from build123d import *

# Parameters (mm, degrees)
F1_DEPTH = 63.5
F0_W     = 25.4
F0_H     = 19.05
F2_DEPTH = 25.4
F3_DEPTH = 7.9375
F5_R     = 6.35


with BuildPart() as f1:
    # F0 (on Front) → F1 (new body, symmetric)
    with BuildSketch(Plane.XZ):
        Polygon((41.275, -9.525), (41.275, 9.525), (22.225, 9.525), (-41.275, 9.525), (-41.275, -9.525), align=None)
    extrude(amount=F1_DEPTH, both=True)

    # F0 (on Front) → F2 (join, symmetric)
    with BuildSketch(Plane.XZ):
        with BuildLine():
            Line((22.225, 9.525), (41.275, 9.525))
            Line((41.275, 9.525), (41.275, 27.0002))
            ThreePointArc((41.275, 27.0002), (45.92468, 38.22552), (57.15, 42.8752))
            Line((57.15, 42.8752), (60.325, 42.8752))
            Line((60.325, 42.8752), (60.325, 61.9252))
            Line((60.325, 61.9252), (57.15, 61.9252))
            ThreePointArc((57.15, 61.9252), (32.454296, 51.695904), (22.225, 27.0002))
            Line((22.225, 27.0002), (22.225, 9.525))
        make_face()
        with Locations((73.025, 52.4002)):
            Rectangle(F0_W, F0_H)
    extrude(amount=F2_DEPTH, both=True)

    # F0 (on Front) → F3 (join, symmetric)
    with BuildSketch(Plane.XZ):
        with BuildLine():
            Line((-41.275, 9.525), (22.225, 9.525))
            Line((22.225, 9.525), (22.225, 27.0002))
            ThreePointArc((22.225, 27.0002), (32.454296, 51.695904), (57.15, 61.9252))
            add(Edge.make_bspline(
                [(-41.275, 9.525), (-25.040152, 44.883206), (20.634502, 62.09904), (57.15, 61.9252)],
                knots=[0, 0, 0, 0, 111.504536, 111.504536, 111.504536, 111.504536], degree=3))
        make_face()
    extrude(amount=F3_DEPTH, both=True)

    # F0 (on Front) → F4 (revolve)
    with BuildSketch(Plane.XZ):
        Polygon((85.725, 42.8752), (60.325, 42.8752), (60.325, 38.1), (111.125, 38.1), (111.125, 66.675), (60.325, 66.675), (60.325, 61.9252), (85.725, 61.9252), align=None)
    revolve(axis=Axis((60.325, 0, 52.3875), (0, 0, -1)))

    # F5
    f5_edges = [f1.edges().sort_by_distance(p)[0] for p in [
        (41.275, -63.5, 0),
        (-41.275, -63.5, 0),
        (-41.275, 63.5, 0),
        (41.275, 63.5, 0),
    ]]
    fillet(f5_edges, radius=F5_R)


solid = f1.part
CAD build for the part. Positions are in the model's coordinates, mm. A direction names the side the tool comes from. Give positions to 0.01 mm unless a question says otherwise; leave off trailing zeros. Write each loop counter-clockwise with the first axis right and the second up, starting at its lowest first coordinate (ties: lowest second). Pieces come first, ordered by that corner, then holes. Notation, with made-up numbers: M -32.5,38 L 19.5,38 A27 ccw 19.5,58 Z; hole C -38,-1.75 d6. An arc over 180 degrees is marked long. Put each result on its own line as item: value. Start each with the question number.
(1) Band-saw the part on A-A, the plane y = 40. Write the cut outline in (x, z) (3 decimals).
(2) Band-saw the part on C-C, the plane x = 15. Write the cut outline in (y, z) (1 decimal).
(3) Probe L1, parallel to X at y = 47.5, z = 5 (3 decimals); L2, parallel to Y at x = 37, z = 59.5; L3, parallel to Z at x = 13.5, y = 57 (3 decimals). List the from-to ranges inside material, lowest first.
(4) Band-saw the part on D-D, the plane y = -55. Write the cut outline in (x, z) (3 decimals), and give its area (3 significant figures).
(5) Band-saw the part on B-B, the plane z = 6. Write the cut outline in (x, y) (3 decimals), and give its area (3 significant figures).
(6) Mould opens along Z. For faces 1 (the face through (41.275, -1, 4)), 2 (the face through (34.93, -0.51, 60.71)), 3 (the face through (41, 7.938, 59)), 4 (the face through (42.418, -0.356, 32.914)) say: +Z half, -Z half, draft (parallel to the pull), parting line (faces both ways), or undercut.
(7) Which spindle directions (+Z, -Z, +X, -X, +Y, -Y) get a long thin tool onto all of the face, cutting with end or side? Do faces 5 (the face through (1, 35, 9.525)), 6 (the face through (31, -25.4, 24)), 7 (the face through (49, 0, 61.925)). Say none if no direction does.
(8) Flat gauge pins, fed straight in: pin 1 Ø8 at (x, z) = (94.5, 47) entering from +Y; pin 2 Ø19 at (x, z) = (37, 28.5) entering from +Y; pin 3 Ø4 at (x, z) = (43, 56.5) entering from -Y; pin 4 Ø2 at (x, y) = (89.5, -43) entering from +Z. Where does each tip first touch, or does it go through?
Response values:
1. outline: M -41.275,-9.525 L 41.275,-9.525 L 41.275,9.525 L -41.275,9.525 Z; M 29.01,38.1 L 91.64,38.1 L 91.64,66.675 L 29.01,66.675 Z
2. outline: M -63.5,-9.5 L 63.5,-9.5 L 63.5,9.5 L 7.9,9.5 L 7.9,38.1 L 22.9,38.1 L 22.9,66.7 L -22.9,66.7 L -22.9,38.1 L -7.9,38.1 L -7.9,9.5 L -63.5,9.5 Z
3. L1: x = -41.275 to 41.275
3. L2: y = -45.13 to -10.06, -7.94 to 7.94, 10.06 to 45.13
3. L3: z = -9.525 to 9.525
4. outline: M -41.275,-9.525 L 41.275,-9.525 L 41.275,9.525 L -41.275,9.525 Z
4. area: 1,570 mm2
5. outline: M -41.275,-57.15 A6.35 ccw -34.925,-63.5 L 34.925,-63.5 A6.35 ccw 41.275,-57.15 L 41.275,57.15 A6.35 ccw 34.925,63.5 L -34.925,63.5 A6.35 ccw -41.275,57.15 Z
5. area: 10,400 mm2
6. face 1: draft
6. face 2: undercut
6. face 3: undercut
6. face 4: -Z half
7. face 5: -X, +Y
7. face 6: +X, -X, -Y
7. face 7: none
8. pin 1: stops at y = 40.87
8. pin 2: stops at y = 25.4
8. pin 3: stops at y = -48.43
8. pin 4: passes through
